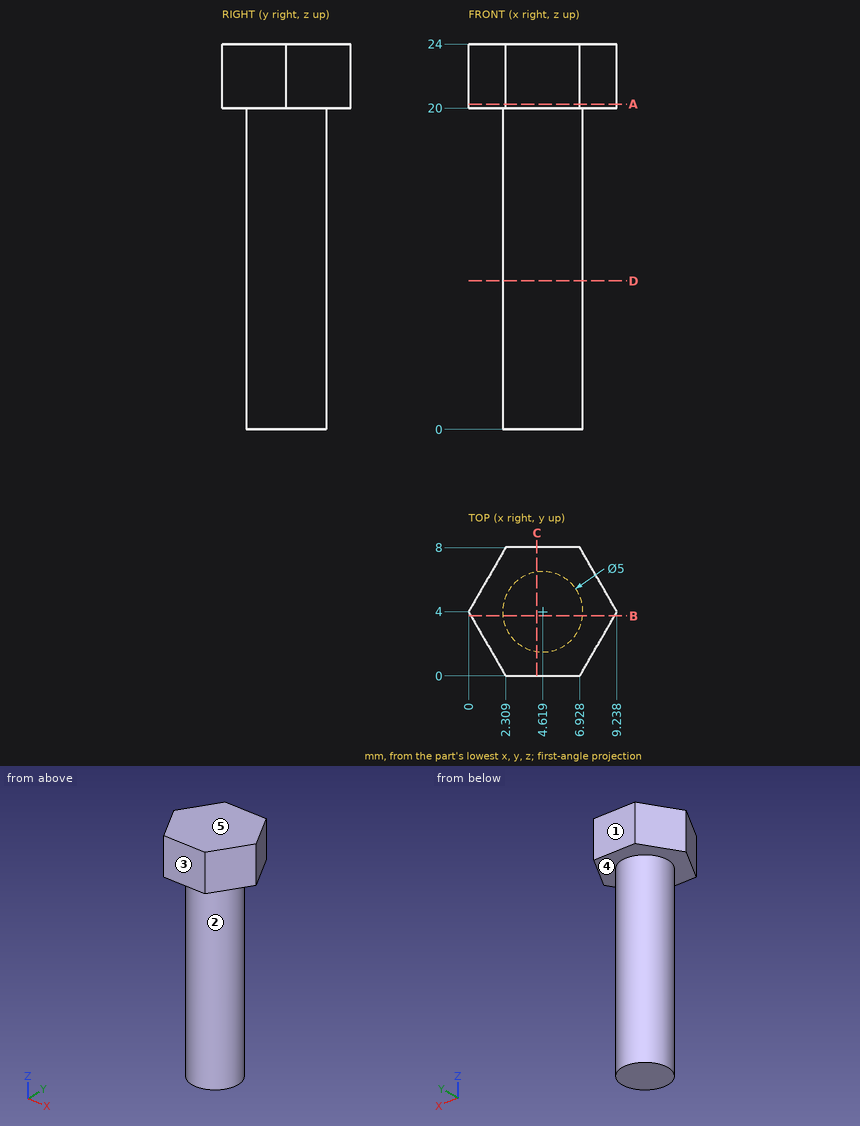
Study the drawing (mm; zero at the part's minimum x, y, z) and answer. A direction names the side the tool comes from. Coordinates: 2 decimals unless noted, no trailing zeros. Order: outer loops, then holes, each group sorted by start corner. A loop starts at its lowest first (then second) coordinate and runs counter-clockwise, first axis right, second up. Notation, with made-up numbers: M 85.25,18 L 113.25,18 A14 ccw 113.25,29 Z; hole C -31.75,81 d1. An arc over 180 degrees is marked long. Answer as a JSON object with one key per item and string values. Group by question number.
1. A tool of negligible diameter and unlimited length cuts with its end or side. For the marked faces 1 and 2, from which of +Z, -Z, +X, -X, +Y, -Y can it reach the whole face along a straight path? Write none if from no direction.
2. Determine the mould class of the marked faces 3, 4 and 5 for opening direction Z: released by +Z, released by -Z, zero draft, split by the parting line, or undercut.
3. Straight lines are drawn through the part: line 1 (Z direction, x = 8, y = 6); line 2 (Y direction, x = 4.5, z = 9.5); line 3 (X direction, y = 4.75, z = 23) (1 decimal). For each, find the intervals that lie inside material, in ascending order.
4. Flat-ended cylindrical pins translate along their axes: P1, Ø4, axis at y = 2, z = 3.5, coming from the -X side; P2, Ø1.5, axis at x = 7.5, z = 15.5, coming from the +Y side (1 decimal); P3, Ø1.5, axis at y = 2.5, z = 11.5, coming from the -X side. Find the tip coordinate at first contact, or state that the pin passes through.
5. Section B-B on y = 3.75 is taken. Write down the section's boundary in (x, z) (1 decimal), then the cut area to 3 significant figures.
6. Section A-A on z = 20.25 is taken. Write down the section's boundary in (x, y).
7. Section D-D on z = 9.25 is taken. Write down the section's boundary in (x, y).
8. Section C-C on x = 4.25 is taken. Write down the section's boundary in (y, z).
Values follow:
{
 "1": {"face 1": "+Z, -Z, +X, -X, +Y", "face 2": "-Z"},
 "2": {"face 3": "zero draft", "face 4": "released by -Z", "face 5": "released by +Z"},
 "3": {"line 1": "20 to 24", "line 2": "1.5 to 6.5", "line 3": "0.4 to 8.8"},
 "4": {"P1": "x = 2.12", "P2": "y = 5.3", "P3": "x = 2.23"},
 "5": {"outline": "M 0.1,20 L 2.1,20 L 2.1,0 L 7.1,0 L 7.1,20 L 9.1,20 L 9.1,24 L 0.1,24 Z", "area": "135 mm2"},
 "6": {"outline": "M 0,4 L 2.31,0 L 6.93,0 L 9.24,4 L 6.93,8 L 2.31,8 Z"},
 "7": {"outline": "C 4.62,4 d5"},
 "8": {"outline": "M 0,20 L 1.53,20 L 1.53,0 L 6.47,0 L 6.47,20 L 8,20 L 8,24 L 0,24 Z"}
}
